Geometry: final body of the model. Coordinates: model frame, mm. Face numbers are marked on the shaded views. A direction names the side the tool comes from. Round coordinates to 2 decimals unless told otherwise and drop trailing zeros. Loops run counter-clockwise (first coordinate to the right, second up) from the corner with the lowest first, then second, coordinate; pieces in that order, holes last. Notation, with made-up numbers: M 74.25,80 L 100.25,80 A26 cw 100.25,116 Z; hole C -29,48.25 d7. An arc over 180 degrees is marked long. Return JSON: item names as keys, results as strings.
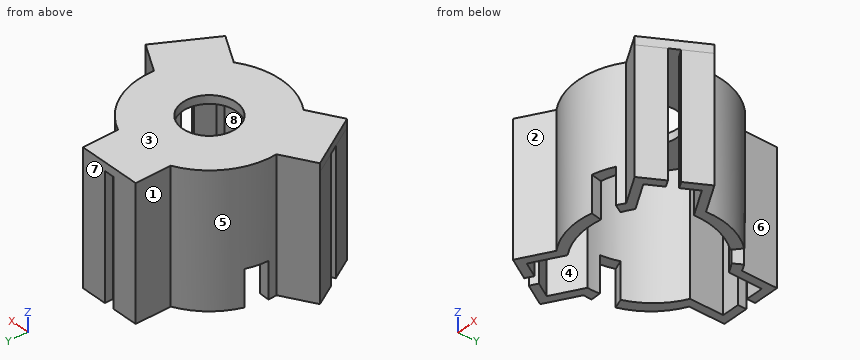
from build123d import *

# Parameters (mm, degrees)
SALIENTE_EXTRUIR1_DEPTH = 0.8
SALIENTE_EXTRUIR2_START = 12
SALIENTE_EXTRUIR2_DEPTH = 12
CROQUIS3_R              = 2.6
CORTAR_EXTRUIR1_DEPTH   = 0.8
CORTAR_EXTRUIR2_DEPTH   = 3.5


with BuildPart() as part:
    # Croquis1 → Saliente-Extruir1 (new body)
    with BuildSketch(Plane.XY):
        with BuildLine():
            Line((-64.04061015, 19.417127137), (-64.04061015, 22.824622624))
            Line((-64.04061015, 22.824622624), (-58.04061015, 22.824622624))
            Line((-58.04061015, 22.824622624), (-58.04061015, 19.417127137))
            ThreePointArc((-58.04061015, 19.417127137), (-54.978432324, 16.592571816), (-54.063384575, 12.528370368))
            Line((-54.063384575, 12.528370368), (-51.11240692, 10.824622624))
            Line((-51.11240692, 10.824622624), (-54.11240692, 5.628470201))
            Line((-54.11240692, 5.628470201), (-57.063384575, 7.332217945))
            ThreePointArc((-57.063384575, 7.332217945), (-61.04061015, 6.092571816), (-65.017835725, 7.332217945))
            Line((-65.017835725, 7.332217945), (-67.96881338, 5.628470201))
            Line((-67.96881338, 5.628470201), (-70.96881338, 10.824622624))
            Line((-70.96881338, 10.824622624), (-68.017835725, 12.528370368))
            ThreePointArc((-68.017835725, 12.528370368), (-67.102787977, 16.592571816), (-64.04061015, 19.417127137))
        make_face()
    extrude(amount=SALIENTE_EXTRUIR1_DEPTH)

    # Croquis2 → Saliente-Extruir2 (add)
    with BuildSketch(Plane(origin=(0, 0, 0), x_dir=(-1, 0, 0), z_dir=(0, 0, -1)).offset(SALIENTE_EXTRUIR2_START)):
        with BuildLine():
            Line((69.71881338, 8.659559114), (70.96881338, 10.824622624))
            Line((70.96881338, 10.824622624), (68.017835725, 12.528370368))
            ThreePointArc((68.017835725, 12.528370368), (67.102787977, 16.592571816), (64.04061015, 19.417127137))
            Line((64.04061015, 19.417127137), (64.04061015, 22.824622624))
            Line((64.04061015, 22.824622624), (61.54061015, 22.824622624))
            Line((61.54061015, 22.824622624), (61.54061015, 22.022889547))
            Line((61.54061015, 22.022889547), (63.24061015, 22.022889547))
            Line((63.24061015, 22.022889547), (63.24061015, 18.822889547))
            ThreePointArc((63.24061015, 18.822889547), (66.17949039, 16.05878973), (67.104711765, 12.131802301))
            Line((67.104711765, 12.131802301), (69.875993057, 10.531802301))
            Line((69.875993057, 10.531802301), (69.025993057, 9.059559114))
            Line((69.025993057, 9.059559114), (69.71881338, 8.659559114))
        make_face()
        with BuildLine():
            Line((65.017835725, 7.332217945), (67.96881338, 5.628470201))
            Line((67.96881338, 5.628470201), (69.21881338, 7.793533711))
            Line((69.21881338, 7.793533711), (68.524492169, 8.194400249))
            Line((68.524492169, 8.194400249), (67.674492169, 6.722157062))
            Line((67.674492169, 6.722157062), (64.903210877, 8.322157062))
            ThreePointArc((64.903210877, 8.322157062), (61.039990097, 7.159062025), (57.176508535, 8.321290524))
            Line((57.176508535, 8.321290524), (54.405227243, 6.721290524))
            Line((54.405227243, 6.721290524), (53.555227243, 8.193533711))
            Line((53.555227243, 8.193533711), (52.86240692, 7.793533711))
            Line((52.86240692, 7.793533711), (54.11240692, 5.628470201))
            Line((54.11240692, 5.628470201), (57.063384575, 7.332217945))
            ThreePointArc((57.063384575, 7.332217945), (61.04061015, 6.092571816), (65.017835725, 7.332217945))
        make_face()
        with BuildLine():
            Line((54.063384575, 12.528370368), (51.11240692, 10.824622624))
            Line((51.11240692, 10.824622624), (52.36240692, 8.659559114))
            Line((52.36240692, 8.659559114), (53.056728131, 9.060425653))
            Line((53.056728131, 9.060425653), (52.206728131, 10.532668839))
            Line((52.206728131, 10.532668839), (54.978009423, 12.132668839))
            ThreePointArc((54.978009423, 12.132668839), (55.902349964, 16.059863694), (58.84061015, 18.824622624))
            Line((58.84061015, 18.824622624), (58.84061015, 22.024622624))
            Line((58.84061015, 22.024622624), (60.54061015, 22.024622624))
            Line((60.54061015, 22.024622624), (60.54061015, 22.824622624))
            Line((60.54061015, 22.824622624), (58.04061015, 22.824622624))
            Line((58.04061015, 22.824622624), (58.04061015, 19.417127137))
            ThreePointArc((58.04061015, 19.417127137), (54.978432324, 16.592571816), (54.063384575, 12.528370368))
        make_face()
    extrude(amount=-SALIENTE_EXTRUIR2_DEPTH)

    # Croquis3 → Cortar-Extruir1 (cut)
    with BuildSketch(Plane(origin=(0, 0, 0), x_dir=(-1, 0, 0), z_dir=(0, 0, -1))):
        with Locations((61.04061015, 13.092571816)):
            Circle(CROQUIS3_R)
    extrude(amount=-CORTAR_EXTRUIR1_DEPTH, mode=Mode.SUBTRACT)

    # Croquis4 → Cortar-Extruir2 (cut)
    with BuildSketch(Plane(origin=(0, 0, -12), x_dir=(-1, 0, 0), z_dir=(0, 0, -1))):
        with BuildLine():
            Line((57.837187447, 18.214022309), (57.328521133, 19.027249156))
            ThreePointArc((57.328521133, 19.027249156), (56.502144155, 18.421955122), (55.772953312, 17.70253835))
            Line((55.772953312, 17.70253835), (56.572877184, 17.024384005))
            ThreePointArc((56.572877184, 17.024384005), (57.168010519, 17.658548761), (57.837187447, 18.214022309))
        make_face()
        with BuildLine():
            Line((67.077627732, 13.30609201), (68.036235998, 13.339996536))
            ThreePointArc((68.036235998, 13.339996536), (67.925224476, 14.358307009), (67.666786697, 15.34951319))
            Line((67.666786697, 15.34951319), (66.679525872, 14.995835968))
            ThreePointArc((66.679525872, 14.995835968), (66.931161993, 14.163353003), (67.077627732, 13.30609201))
        make_face()
        with BuildLine():
            Line((58.207015271, 7.757601131), (57.757073319, 6.910469757))
            ThreePointArc((57.757073319, 6.910469757), (58.694461819, 6.497453318), (59.682090441, 6.22566391))
            Line((59.682090441, 6.22566391), (59.869427395, 7.257495476))
            ThreePointArc((59.869427395, 7.257495476), (59.022657939, 7.455813685), (58.207015271, 7.757601131))
        make_face()
    extrude(amount=-CORTAR_EXTRUIR2_DEPTH, mode=Mode.SUBTRACT)


solid = part.part
Q1. Reachability of the marked faces 1, 2, 3, 4 and 5 from +Z, -Z, +X, -X, +Y, -Y: full face, straight path, thin tool, end or side. Return the list, or none.
Determined:
{"face 1": "+Z, -Z, -X, +Y", "face 2": "+Z, -Z, -Y", "face 3": "+Z, +X, -X, +Y, -Y", "face 4": "-Z", "face 5": "+Z, -Z, -X"}
Q2. Section query B-B (z = -5.25). State how many separate pieces and enclosed holes the cut face has, plus the area to 3 significant figures.
Determined:
{"separate pieces": "3", "enclosed holes": "0", "area": "51.0 mm^2"}
Q3. Pull-direction query (Y, two-part tool) for the marked faces 6, 7 and 8; classes: pulls with the +Y half, pulls with the -Y half, needs draft (parallel to the pull), parting line crosses it, or undercut.
Determined:
{"face 6": "needs draft", "face 7": "pulls with the +Y half", "face 8": "undercut"}
Q4. Material intervals for L1, parallel to X at y = 7, z = -9; L2, parallel to X at y = 20, z = -0.5; L3, parallel to Z at x = -65.25, y = 14.5, sorted ascending.
Determined:
{"L1": "x = -68.76 to -67.83, -67.19 to -65.59, -64.49 to -59.82, -57.8 to -57.59, -56.49 to -54.89, -54.24 to -53.32", "L2": "x = -64.04 to -63.24, -58.84 to -58.04", "L3": "z = 0 to 0.8"}
Q5. Section query D-D (y = 11.75). Output: boundary loops of the cut face in (x, z), plus the area to 3 significant figures.
Determined:
{"outline": "M -69.37,-12 L -67.77,-12 L -67.77,0 L -63.27,0 L -63.27,0.8 L -69.37,0.8 Z; M -58.81,0 L -54.32,0 L -54.32,-12 L -52.72,-12 L -52.72,0.8 L -58.81,0.8 Z", "area": "48.2 mm^2"}
Q6. Pin query (flat end, axial travel): pin 1 (10 mm diameter, centred on x = -55.5, y = 19.5, fed in from +Z); pin 2 (3.5 mm diameter, centred on y = 21, z = -8.5, fed in from +X); pin 3 (5 mm diameter, centred on x = -62, y = 12.5, fed in from -Z); pin 4 (0.5 mm diameter, centred on x = -62.5, z = -5.5, fed in from -Y). Return the tip coordinate at first contact, or that it passes through.
Determined:
{"pin 1": "stops at z = 0.8", "pin 2": "stops at x = -57.71", "pin 3": "stops at z = 0", "pin 4": "stops at y = 6.2"}
Q7. Section query C-C (x = -64.5). Output: boundary loops of the cut face in (y, z), plus the area to 3 significant figures.
Determined:
{"outline": "M 7.01,-12 L 8.07,-12 L 8.07,0 L 18.02,0 L 18.02,-12 L 19.18,-12 L 19.18,0.8 L 7.01,0.8 Z", "area": "36.5 mm^2"}
Q8. Section query A-A (y = 13.75). Output: boundary loops of the cut face in (x, z), plus the area to 3 significant figures.
Determined:
{"outline": "M -68.01,-8.5 L -67.02,-8.5 L -67.02,0 L -63.56,0 L -63.56,0.8 L -68.01,0.8 Z; M -58.53,0 L -55.07,0 L -55.07,-12 L -54.07,-12 L -54.07,0.8 L -58.53,0.8 Z", "area": "27.5 mm^2"}
